Can you work these out from the model? Positions are in its coordinate system, mm. A direction names the side the tool comes from. Give positions to 0.01 mm unless a question says otherwise; leave off trailing zeros. Write each loop counter-clockwise with the first axis right and the second up, starting at its lowest first coordinate (ties: lowest second). Pieces come first, ordered by that corner, then holes. Notation, with made-up numbers: M 5.5,3 L 47.5,3 A19 cw 47.5,28 Z; hole C -6.75,-22 d6. An arc over 180 degrees is marked long. Write each question's results on one line, items separated by ' | '.
from build123d import *

# Parameters (mm, degrees)
F0_W     = 22.5392356515
F0_H     = 17.0982331038
F0_W_2   = 21.3571861386
F0_H_2   = 32.321177423
F2_DEPTH = 51.5995789319
F4_SIZE  = 5.08


with BuildPart() as f1:
    # F0 (on Front) → F1 (revolve)
    with BuildSketch(Plane.XZ):
        with Locations((11.2696178257, 33.5941463709)):
            Rectangle(F0_W, F0_H)
        with Locations((33.2178287208, 33.5941463709)):
            Rectangle(F0_W_2, F0_H)
        with Locations((11.2696178257, 58.3038516343)):
            Rectangle(F0_W, F0_H_2)
    revolve(axis=Axis((22.569514811, 0, 0), (1, 0, 0)))

    # F2 (add): a face of the model
    f2_faces = [f1.faces().sort_by_distance(p)[0] for p in [
        (0, 0, -72.3582679167),
    ]]
    extrude(f2_faces, amount=F2_DEPTH)

    # F4
    f4_edges = [f1.edges().sort_by_distance(p)[0] for p in [
        (43.896422, 0, -42.143263),
    ]]
    chamfer(f4_edges, length=F4_SIZE)


solid = f1.part
Item 1: I want a section at A-A, the plane z = 0. Please give me the cut outline in (x, y).
Geometry says:
outline: M -51.6,-74.46 L 22.54,-74.46 L 22.54,-42.14 L 38.82,-42.14 L 43.9,-37.06 L 43.9,-25.05 L -51.6,-25.05 Z; M -51.6,25.05 L 43.9,25.05 L 43.9,37.06 L 38.82,42.14 L 22.54,42.14 L 22.54,74.46 L -51.6,74.46 Z
Item 2: For faces 1 (the face through (22.539, 32, -32)), 2 (the face through (-14, 45.3, -59.1)), which set-ups out of +Z, -Z, +X, -X, +Y, -Y let a thin tool reach every point of the face, with its end or its side?
Geometry says:
face 1: +X | face 2: +X, -X
Item 3: If I drill on line 1 (Z direction, x = -18, y = 0); line 2 (X direction, y = 41, z = 27.5), over which ranges is the centre line in solid material (lowest first)? Write a range as from..to.
Geometry says:
line 1: z = -74.46..-25.05, 25.05..74.46 | line 2: x = -51.6..22.54
Item 4: I want a section at C-C, the plane x = 24.5. Please give me the cut outline in (y, z).
Geometry says:
outline: C 0,0 d84.29; hole C 0,0 d50.09
Item 5: I want a section at D-D, the plane x = -17.5. Please give me the cut outline in (y, z).
Geometry says:
outline: C 0,0 d148.93; hole C 0,0 d50.09
Item 6: Thinking about a two-plate mould opening in Y: for faces 3 (the face through (30.56, 41.14, -9.14)), 4 (the face through (-51.6, 32, -1)), 5 (the face through (-3.183, 15.24, -19.875)), which applies, +Y half, -Y half, draft (parallel to the pull), parting line (faces both ways), or undercut?
Geometry says:
face 3: parting line | face 4: draft | face 5: undercut
Item 7: I'm going to push flat-ended pins straight in: pin 1 (3 mm diameter, centred on x = 9.5, y = 49.5, fed in from +Z); pin 2 (10 mm diameter, centred on x = -1, z = 36, fed in from -Y); pin 3 (4 mm diameter, centred on x = -11, z = 51, fed in from -Y). Where does each tip first touch, or does it pass through?
Geometry says:
pin 1: stops at z = 56.93 | pin 2: stops at y = -67.7 | pin 3: stops at y = -56.07
